Verification items for this drawing (mm, ordinates from the low corner). A direction names the side the tool comes from. Round coordinates to 2 decimals unless told otherwise and drop trailing zeros. Order: outer loops, then holes, each group sorted by start corner. A loop starts at its lowest first (then second) coordinate and runs counter-clockwise, first axis right, second up. Notation, with made-up numbers: M -1.5,-3 L 40.5,-3 A7 cw 40.5,7 Z; hole C 63.25,31 d1. An arc over 180 degrees is marked long. One line per item, written item: value. Start each with the question number.
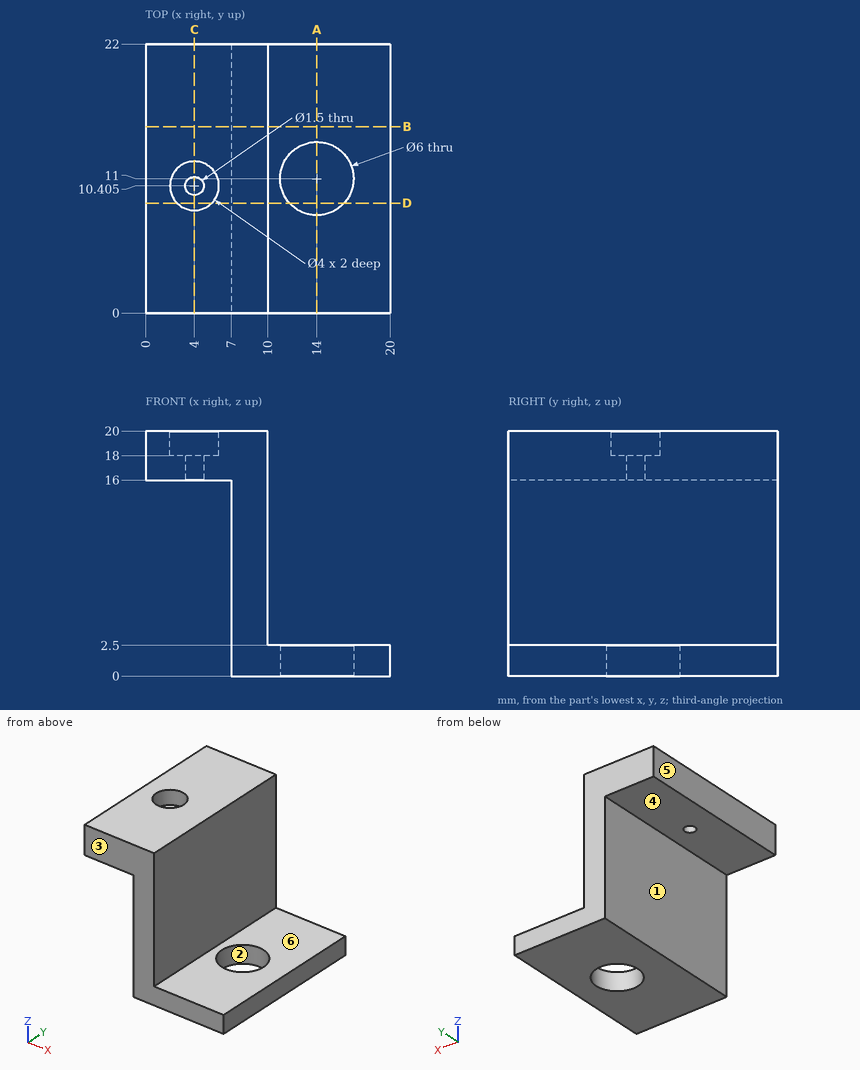
1. Scan lines: line 1 along Y through (x, z) = (4, 17) (1 decimal); line 2 along Z through (x, y) = (16.25, 5.75); line 3 along X through (y, z) = (14.5, 12). Record each from-to range of solid material in increasing order.
2. Draft check along Y on the marked faces 1, 2 and 3. Enter one of: released by +Y, released by -Y, zero draft, split by the parting line, or undercut.
3. Section check A-A (x = 14). Record the cut outline in (y, z).
4. Section check C-C (x = 4). Record the cut outline in (y, z) (1 decimal).
5. Tool access check on the marked faces 4, 5 and 6. Record the directions out of +Z, -Z, +X, -X, +Y, -Y that give a thin tool (end or side, any length) a straight path to the whole face; none if there is none.
6. Section check D-D (y = 9). Record the cut outline in (x, z).
7. Depth check by flat-ended pin: pin 1 (5 mm diameter, centred on y = 10, z = 6, fed in from -X); pin 2 (6 mm diameter, centred on x = 15.5, y = 8, fed in from +Z); pin 3 (2.5 mm diameter, centred on x = 4, y = 10.41, fed in from +Z); pin 4 (5 mm diameter, centred on x = 14, y = 11, fed in from -Z). Enter the tip coordinate at first touch or a pass-through.
8. Section check B-B (y = 15.25). Record the cut outline in (x, z), and give its area (3 significant figures).
Geometry check:
1. line 1: y = 0 to 9.7, 11.2 to 22
1. line 2: z = 0 to 2.5
1. line 3: x = 7 to 10
2. face 1: zero draft
2. face 2: undercut
2. face 3: released by -Y
3. outline: M 0,0 L 8,0 L 8,2.5 L 0,2.5 Z; M 14,0 L 22,0 L 22,2.5 L 14,2.5 Z
4. outline: M 0,16 L 9.7,16 L 9.7,18 L 8.4,18 L 8.4,20 L 0,20 Z; M 11.2,16 L 22,16 L 22,20 L 12.4,20 L 12.4,18 L 11.2,18 Z
5. face 4: -Z, -X, +Y, -Y
5. face 5: +Z, -Z, -X, +Y, -Y
5. face 6: +Z, +X, +Y, -Y
6. outline: M 0,16 L 7,16 L 7,0 L 11.76,0 L 11.76,2.5 L 10,2.5 L 10,20 L 5.42,20 L 5.42,18 L 2.58,18 L 2.58,20 L 0,20 Z; M 16.24,0 L 20,0 L 20,2.5 L 16.24,2.5 Z
7. pin 1: stops at x = 7
7. pin 2: stops at z = 2.5
7. pin 3: stops at z = 18
7. pin 4: passes through
8. outline: M 0,16 L 7,16 L 7,0 L 20,0 L 20,2.5 L 10,2.5 L 10,20 L 0,20 Z
8. area: 113 mm²
